from build123d import *

# Parameters (mm, degrees)
SALIENTE_EXTRUIR1_DEPTH = 6.35
CROQUIS2_R              = 6.35
CORTAR_EXTRUIR1_DEPTH   = 5
CROQUIS3_R              = 3.8
CORTAR_EXTRUIR2_DEPTH   = 2.35
CROQUIS4_R              = 3.175
CORTAR_EXTRUIR3_DEPTH   = 5
CROQUIS5_R              = 1.5
CORTAR_EXTRUIR4_DEPTH   = 5
CROQUIS6_R              = 1.5
CORTAR_EXTRUIR5_DEPTH   = 5
CROQUIS7_R              = 6.35
CORTAR_EXTRUIR6_DEPTH   = 5
CROQUIS8_R              = 3.5
CORTAR_EXTRUIR7_DEPTH   = 5
CROQUIS9_R              = 1.5
CORTAR_EXTRUIR8_DEPTH   = 5


with BuildPart() as part:
    # Croquis1 → Saliente-Extruir1 (new body)
    with BuildSketch(Plane.XY):
        with BuildLine():
            Line((10, 42.5), (10, -42.5))
            ThreePointArc((10, -42.5), (0, -52.5), (-10, -42.5))
            Line((-10, -42.5), (-10, 42.5))
            ThreePointArc((-10, 42.5), (0, 52.5), (10, 42.5))
        make_face()
    extrude(amount=SALIENTE_EXTRUIR1_DEPTH)

    # Croquis2 → Cortar-Extruir1 (cut)
    with BuildSketch(Plane.XY.offset(6.35)):
        with Locations((0, 42.5)):
            Circle(CROQUIS2_R)
    extrude(amount=-CORTAR_EXTRUIR1_DEPTH, mode=Mode.SUBTRACT)

    # Croquis3 → Cortar-Extruir2 (cut, through all)
    with BuildSketch(Plane.XY.offset(1.35)):
        with Locations((0, 42.5)):
            Circle(CROQUIS3_R)
    extrude(amount=-CORTAR_EXTRUIR2_DEPTH, mode=Mode.SUBTRACT)

    # Croquis4 → Cortar-Extruir3 (cut)
    with BuildSketch(Plane.XY.offset(6.35)):
        with Locations((5.175, 30.5)):
            Circle(CROQUIS4_R)
        with Locations((-5.175, 30.5)):
            Circle(CROQUIS4_R)
    extrude(amount=-CORTAR_EXTRUIR3_DEPTH, mode=Mode.SUBTRACT)

    # Croquis5 → Cortar-Extruir4 (cut)
    with BuildSketch(Plane.XY.offset(1.35)):
        with Locations((-5.175, 30.5)):
            Circle(CROQUIS5_R)
        with Locations((5.175, 30.5)):
            Circle(CROQUIS5_R)
    extrude(amount=-CORTAR_EXTRUIR4_DEPTH, mode=Mode.SUBTRACT)

    # Croquis6 → Cortar-Extruir5 (cut)
    with BuildSketch(Plane(origin=(10, 0, 0), x_dir=(0, 0, -1), z_dir=(1, 0, 0))):
        with Locations((-3.175, 42.5)):
            Circle(CROQUIS6_R)
    extrude(amount=-CORTAR_EXTRUIR5_DEPTH, mode=Mode.SUBTRACT)

    # Croquis7 → Cortar-Extruir6 (cut)
    with BuildSketch(Plane(origin=(0, 0, 0), x_dir=(-1, 0, 0), z_dir=(0, 0, -1))):
        with Locations((0, -42.5)):
            Circle(CROQUIS7_R)
    extrude(amount=-CORTAR_EXTRUIR6_DEPTH, mode=Mode.SUBTRACT)

    # Croquis8 → Cortar-Extruir7 (cut)
    with BuildSketch(Plane(origin=(0, 0, 5), x_dir=(-1, 0, 0), z_dir=(0, 0, -1))):
        with Locations((0, -42.5)):
            Circle(CROQUIS8_R)
    extrude(amount=-CORTAR_EXTRUIR7_DEPTH, mode=Mode.SUBTRACT)

    # Croquis9 → Cortar-Extruir8 (cut)
    with BuildSketch(Plane(origin=(10, 0, 0), x_dir=(0, 0, -1), z_dir=(1, 0, 0))):
        with Locations((-3.175, -42.5)):
            Circle(CROQUIS9_R)
    extrude(amount=-CORTAR_EXTRUIR8_DEPTH, mode=Mode.SUBTRACT)


solid = part.part
Verification items for the finished model (mm, model axes). A direction names the side the tool comes from. Coordinates: 2 decimals unless noted, no trailing zeros. Order: outer loops, then holes, each group sorted by start corner. A loop starts at its lowest first (then second) coordinate and runs counter-clockwise, first axis right, second up.
Item 1: Section check B-B, the plane y = 30.5. Enter the section's corners in (x, z) (3 decimals), then the cut area to 3 significant figures.
Filled in:
outline: (-10, 0) - (-6.675, 0) - (-6.675, 1.35) - (-8.35, 1.35) - (-8.35, 6.35) - (-10, 6.35) - close; (-3.675, 0) - (3.675, 0) - (3.675, 1.35) - (2, 1.35) - (2, 6.35) - (-2, 6.35) - (-2, 1.35) - (-3.675, 1.35) - close; (6.675, 0) - (10, 0) - (10, 6.35) - (8.35, 6.35) - (8.35, 1.35) - (6.675, 1.35) - close
area: 55.4 mm2
Item 2: Section check A-A, the plane x = 0. Enter the section's corners in (y, z), then the cut area to 3 significant figures.
Filled in:
outline: (-52.5, 0) - (-48.85, 0) - (-48.85, 5) - (-46, 5) - (-46, 6.35) - (-52.5, 6.35) - close; (-39, 5) - (-36.15, 5) - (-36.15, 0) - (38.7, 0) - (38.7, 1.35) - (36.15, 1.35) - (36.15, 6.35) - (-39, 6.35) - close; (46.3, 0) - (52.5, 0) - (52.5, 6.35) - (48.85, 6.35) - (48.85, 1.35) - (46.3, 1.35) - close
area: 520 mm2
Item 3: Depth check by flat-ended pin: pin 1 (2.5 mm diameter, centred on x = -5.175, y = 30.5, fed in from -Z); pin 2 (2.5 mm diameter, centred on y = -42.5, z = 3.175, fed in from +X); pin 3 (3 mm diameter, centred on x = 7, z = 3.5, fed in from +Y); pin 4 (2 mm diameter, centred on x = -4, z = 5.5, fed in from +Y). Enter the tip coordinate at first touch or a pass-through.
Filled in:
pin 1: passes through
pin 2: stops at x = -6.23
pin 3: stops at y = 50.85
pin 4: stops at y = 52.04
Item 4: Access from +Z, -Z, +X, -X, +Y, -Y to the whole of each face (thin tool, end or side, straight path). Record for faces 1 (the face through (-6.057, -40.593, 2.465)), 2 (the face through (8.112, -43.964, 3.5)), 3 (the face through (4.49, 27.4, 3.88)).
Filled in:
face 1: -Z
face 2: +X
face 3: +Z
Item 5: Material ranges on L1, parallel to Z at x = 8.3, y = -42.5 (3 decimals); L2, parallel to Y at x = 4.5, z = 6.25; L3, parallel to Y at x = -0.5, z = 3, recorded low to high.
Filled in:
L1: z = 0 to 1.675, 4.675 to 6.35
L2: y = -51.43 to 27.4, 33.6 to 38.02, 46.98 to 51.43
L3: y = -52.49 to -48.83, -36.17 to 36.17, 48.83 to 52.49
Item 6: Section check C-C, the plane x = 5. Enter the section's corners in (y, z).
Filled in:
outline: (-51.16, 0) - (-46.41, 0) - (-46.41, 5) - (-38.59, 5) - (-38.59, 0) - (29.01, 0) - (29.01, 1.35) - (27.33, 1.35) - (27.33, 6.35) - (-51.16, 6.35) - close; (31.99, 0) - (51.16, 0) - (51.16, 6.35) - (46.41, 6.35) - (46.41, 1.35) - (38.59, 1.35) - (38.59, 6.35) - (33.67, 6.35) - (33.67, 1.35) - (31.99, 1.35) - close
Item 7: Release check for a two-part mould opening along Y. For faces 4 (the face through (0.2, -52.5, 3.1)), 5 (the face through (0, 1, 0)), 6 (the face through (-5.86, 27.4, 3.88)) record: +Y half, -Y half, draft (parallel to the pull), parting line (faces both ways), or undercut.
Filled in:
face 4: -Y half
face 5: draft
face 6: undercut
